```python
from build123d import *

# Parameters (mm, degrees)
SKETCH2_R                = 17.5
BOSS_EXTRUDE2_DEPTH      = 101.6
SKETCH3_R                = 45
BOSS_EXTRUDE3_DEPTH      = 6.35
SKETCH4_R                = 9
CUT_EXTRUDE1_DEPTH       = 95.25
SKETCH5_R                = 14.999999972
CUT_EXTRUDE2_DEPTH       = 96.6
SKETCH6_R                = 2.5
CUT_EXTRUDE3_DEPTH       = 120.885612148
BOSS_EXTRUDE4_DEPTH      = 5
BOSS_EXTRUDE4_DEPTH_BACK = 2
SKETCH8_R                = 2.5
SKETCH9_R                = 3.75
CUT_EXTRUDE4_DEPTH       = 115.553753758
CIRPATTERN1_COUNT        = 3


with BuildPart() as part:
    # Sketch2 → Boss-Extrude2 (new body)
    with BuildSketch(Plane(origin=(0, 0, 0), x_dir=(1, 0, 0), z_dir=(0, 1, 0))):
        with Locations(Location((0, 0, 0), (0, 0, 270))):
            Circle(SKETCH2_R)
    extrude(amount=BOSS_EXTRUDE2_DEPTH)

    # Sketch3 → Boss-Extrude3 (add)
    with BuildSketch(Plane(origin=(0, 0, 0), x_dir=(-1, 0, 0), z_dir=(0, -1, 0))):
        with Locations(Location((0, 0, 0), (0, 0, 90))):
            Circle(SKETCH3_R)
    extrude(amount=-BOSS_EXTRUDE3_DEPTH)

    # Sketch4 → Cut-Extrude1 (cut)
    with BuildSketch(Plane(origin=(0, 0, 0), x_dir=(-1, 0, 0), z_dir=(0, -1, 0))):
        with Locations(Location((0, 0, 0), (0, 0, 90))):
            Circle(SKETCH4_R)
    extrude(amount=-CUT_EXTRUDE1_DEPTH, mode=Mode.SUBTRACT)

    # Sketch5 → Cut-Extrude2 (cut)
    with BuildSketch(Plane(origin=(0, 101.6, 0), x_dir=(1, 0, 0), z_dir=(0, 1, 0))):
        with Locations(Location((0, 0, 0), (0, 0, 270))):
            Circle(SKETCH5_R)
    extrude(amount=-CUT_EXTRUDE2_DEPTH, mode=Mode.SUBTRACT)

    # Sketch6 → Cut-Extrude3 (cut, through all)
    with BuildSketch(Plane(origin=(0, 0, 0), x_dir=(0, 0, -1), z_dir=(1, 0, 0))):
        with Locations(Location((0, 56.35, 0), (0, 0, 180))):
            Circle(SKETCH6_R)
    extrude(amount=CUT_EXTRUDE3_DEPTH, mode=Mode.SUBTRACT)

    # Sketch8 → Boss-Extrude4 (add, two sides: drawn at the far end of the back side and taken through both)
    with BuildSketch(Plane.ZY.offset(-17.5).offset(-BOSS_EXTRUDE4_DEPTH_BACK)):
        Polygon((-5, 53.463248654), (0, 50.576497308), (5, 53.463248654), (5, 59.236751346), (0, 62.123502692), (-5, 59.236751346), align=None)
        with Locations((0, 56.35)):
            Circle(SKETCH8_R, mode=Mode.SUBTRACT)
    extrude(amount=BOSS_EXTRUDE4_DEPTH + BOSS_EXTRUDE4_DEPTH_BACK)

    # Sketch9 → Cut-Extrude4 (cut, through all)
    with BuildSketch(Plane(origin=(0, 6.35, 0), x_dir=(1, 0, 0), z_dir=(0, 1, 0))):
        with Locations(Location((-31.25, 0, 0), (0, 0, 270))):
            Circle(SKETCH9_R)
    cut_extrude4 = extrude(amount=-CUT_EXTRUDE4_DEPTH, mode=Mode.SUBTRACT)

    # CirPattern1: Cut-Extrude4 ×3 about axis
    cirpattern1_axis = Axis((0, 0, 0), (0, 1, 0))
    for i in range(1, CIRPATTERN1_COUNT):
        add(cut_extrude4.rotate(cirpattern1_axis, i * 360 / CIRPATTERN1_COUNT), mode=Mode.SUBTRACT)


solid = part.part
```
Model file for the job. Use its own axes, mm. A direction names the side the tool comes from. Coordinates: 2 decimals unless noted, no trailing zeros. Loops run counter-clockwise (first coordinate to the right, second up) from the corner with the lowest first, then second, coordinate; pieces in that order, holes last. Notation, with made-up numbers: (-32.75, 55) - (21.25, 55) arc R17 ccw to (21.25, 71) - close; hole circle Ø10 at (56.25, 48.5). An arc over 180 degrees is marked (long way). Answer as a JSON object with one key per item and string values. Group by question number.
(1) Two-plate mould, pull along X, no slides. Class faces 5 (the face through (11.964, 3.219, -27.876)), 6 (the face through (1, 6.35, -19)), 7 (the face through (-17.235, 3.131, -41.569)): released by +X, released by -X, zero draft, split by the parting line, or undercut.
(2) Cut at C-C (x = -13). Give the cut face in (y, z).
(3) Probe line 1 along X through (y, z) = (1.55, 0); line 2 along Y through (x, z) = (13.6, 0); line 3 along X through (y, z) = (5.25, 0). List the from-to ranges inside material, lowest first.
(4) Cut at D-D (y = 93.5). Give the cut face in (x, z), then the cut area to 3 significant figures.
(5) Tool access for faces 1 (the face through (18.458, 60.7, -2.465)), 2 (the face through (18.458, 52, 2.465)), 3 (the face through (13.767, 60.7, -2.465)), 4 (the face through (18.458, 60.66, 2.535)): list every direction of +Z, -Z, +X, -X, +Y, -Y with a clear straight run to the whole face (end or side of a thin tool).
(6) Cut at A-A (x = 0). Give the cut face in (y, z).
(7) Cut at B-B (y = 56.35). Give the cut face in (x, z).
(8) Flat gauge pins, fed straight in: pin 1 (4.5 mm diameter, centred on y = 56.35, z = 0, fed in from +X); pin 2 (0.5 mm diameter, centred on x = 13, y = 56, fed in from -Z); pin 3 (3 mm diameter, centred on x = 18.5, y = 55, fed in from +Z). Where does each tip first touch, or does it go through?
Geometry says:
{
 "1": {"face 5": "undercut", "face 6": "zero draft", "face 7": "split by the parting line"},
 "2": {"outline": "(0, -43.08) - (6.35, -43.08) - (6.35, -11.72) - (101.6, -11.72) - (101.6, -7.48) - (5, -7.48) - (5, 7.48) - (101.6, 7.48) - (101.6, 11.72) - (6.35, 11.72) - (6.35, 43.08) - (0, 43.08) - close"},
 "3": {"line 1": "x = -45 to -35, -27.5 to -9, 9 to 45", "line 2": "y = 0 to 5, 50.58 to 53.85, 58.85 to 62.12", "line 3": "x = -45 to -35, -27.5 to -15, 15 to 45"},
 "4": {"outline": "circle Ø35 at (0, 0); hole circle Ø30 at (0, 0)", "area": "255 mm^2"},
 "5": {"face 1": "-Z, +X, +Y", "face 2": "+Z, +X", "face 3": "+Y", "face 4": "+Z, +X, +Y"},
 "6": {"outline": "(0, -45) - (6.35, -45) - (6.35, -17.5) - (101.6, -17.5) - (101.6, -15) - (5, -15) - (5, -9) - (0, -9) - close; (0, 9) - (5, 9) - (5, 15) - (101.6, 15) - (101.6, 17.5) - (6.35, 17.5) - (6.35, 45) - (0, 45) - close"},
 "7": {"outline": "(12.5, -5) - (14.14, -5) arc R15 cw (long way) to (14.14, 5) - (12.5, 5) - (12.5, 2.5) - (19.5, 2.5) - (19.5, 5) - (16.77, 5) arc R17.5 ccw (long way) to (16.77, -5) - (19.5, -5) - (19.5, -2.5) - (12.5, -2.5) - close"},
 "8": {"pin 1": "stops at x = -14.83", "pin 2": "stops at z = -11.99", "pin 3": "stops at z = 5"}
}
